from build123d import *

# Parameters (mm, degrees)
SKETCH1_R           = 28
SKETCH1_R_2         = 15
BOSS_EXTRUDE1_DEPTH = 106
SKETCH4_R           = 28
SKETCH4_R_2         = 15
BOSS_EXTRUDE2_DEPTH = 53
CUT_EXTRUDE2_START  = -106
SKETCH5_R           = 15
CUT_EXTRUDE2_DEPTH  = 106
SCALE1_SCALE        = 0.33


with BuildPart() as part:
    # Sketch1 → Boss-Extrude1 (new body)
    with BuildSketch(Plane(origin=(0, 0, 0), x_dir=(1, 0, 0), z_dir=(0, 1, 0))):
        with Locations(Location((0, 0, 0), (0, 0, 270))):
            Circle(SKETCH1_R)
        with Locations(Location((0, 0, 0), (0, 0, 270))):
            Circle(SKETCH1_R_2, mode=Mode.SUBTRACT)
    extrude(amount=BOSS_EXTRUDE1_DEPTH)

    # Sketch4 → Boss-Extrude2 (add, symmetric)
    with BuildSketch(Plane(origin=(0, 0, 0), x_dir=(0, 0, -1), z_dir=(1, 0, 0))):
        with Locations((38, 53)):
            Circle(SKETCH4_R)
        with Locations((38, 53)):
            Circle(SKETCH4_R_2, mode=Mode.SUBTRACT)
    extrude(amount=BOSS_EXTRUDE2_DEPTH, both=True)

    # Sketch5 → Cut-Extrude2 (cut)
    with BuildSketch(Plane(origin=(53, 0, 0), x_dir=(0, 0, -1), z_dir=(1, 0, 0)).offset(CUT_EXTRUDE2_START)):
        with Locations((38, 53)):
            Circle(SKETCH5_R)
    extrude(amount=CUT_EXTRUDE2_DEPTH, mode=Mode.SUBTRACT)


with BuildPart() as part_1:
    # Scale1: scaled about (-6.4e-07, 52.999995481, -18.972102588)
    add(part.part.scale(SCALE1_SCALE).moved(Location((-4.29e-07, 35.509996972, -12.711308734))))


solid = part_1.part
Build history of the part. All positions in model axes, mm. A direction names the side the tool comes from. Coordinates: 2 decimals unless noted, no trailing zeros. Write each loop counter-clockwise with the first axis right and the second up, starting at its lowest first coordinate (ties: lowest second). Pieces come first, ordered by that corner, then holes.
(1) Cut at C-C on y = 60. List the corners of the cut face in (x, z), and give its area (3 significant figures).
(2) 3-axis set-ups, long thin cutter, end or side, ignore diameter. For faces 4 (the cylindrical face through (0.05, 53.08, -16.01)), 5 (the flat face through (17.49, 49, -29)): which of +Z, -Z, +X, -X, +Y, -Y reach the whole face in a straight line?
(3) Cut at B-B on z = -15. List the corners of the cut face in (x, y).
(4) Cut at A-A on x = 2. List the corners of the cut face in (y, z), and give its area (3 significant figures).
(5) Cut at D-D on x = -7. List the corners of the cut face in (y, z).
(6) Drill centre lines: line 1 (Z direction, x = 0, y = 53); line 2 (Z direction, x = 0, y = 51.5); line 3 (Z direction, x = 5, y = 55.5). Where is each one in solid material? Low to high.
(7) Mould opens along X. For faces 1 (the cylindrical face through (2.78, 52.76, -3.9)), 2 (the cylindrical face through (1.49, 52.76, -7.99)), 3 (the flat face through (-4, 70.49, -9)) say: pulls with the +X half, pulls with the -X half, needs draft (parallel to the pull), parting line crosses it, or undercut.
(8) Pin check, flat tips, straight feed: pin 1 Ø9 at (y, z) = (53, -25.25) entering from +X; pin 2 Ø1.5 at (x, y) = (7, 51.5) entering from -Z; pin 3 Ø11.5 at (x, z) = (0, -12.71) entering from +Y; pin 4 Ø6 at (y, z) = (61, -11.5) entering from -X. Stop position of each tip, or through.
Working result:
1. outline: (-17.49, -31.28) - (17.49, -31.28) - (17.49, -19.22) - (6.56, -19.22) arc R9.24 ccw (long way) to (-6.56, -19.22) - (-17.49, -19.22) - close; hole circle Ø9.9 at (0, -12.71)
1. area: 589 mm2
2. face 4: none
2. face 5: +Z, -Z, +X, +Y, -Y
3. outline: (-8.95, 35.51) - (-4.39, 35.51) - (-4.39, 70.49) - (-8.95, 70.49) - close; (4.39, 35.51) - (8.95, 35.51) - (8.95, 70.49) - (4.39, 70.49) - close
4. outline: (35.51, -21.73) - (44.46, -21.73) arc R9.24 ccw (long way) to (61.54, -21.73) - (70.49, -21.73) - (70.49, -17.24) - (57.6, -17.24) arc R9.24 ccw to (48.4, -17.24) - (35.51, -17.24) - close; (35.51, -8.18) - (70.49, -8.18) - (70.49, -3.69) - (35.51, -3.69) - close; hole circle Ø9.9 at (53, -25.25)
4. area: 443 mm2
5. outline: (35.51, -18.74) - (46.44, -18.74) arc R9.24 ccw (long way) to (59.56, -18.74) - (70.49, -18.74) - (70.49, -6.68) - (35.51, -6.68) - close; hole circle Ø9.9 at (53, -25.25)
6. line 1: z = -34.49 to -30.2, -20.3 to -16.01, -7.76 to -3.47
6. line 2: z = -34.37 to -29.97, -20.53 to -16.13, -7.76 to -3.47
6. line 3: z = -34.15 to -29.52, -20.98 to -4.94
7. face 1: parting line crosses it
7. face 2: undercut
7. face 3: needs draft
8. pin 1: passes through
8. pin 2: stops at z = -34.46
8. pin 3: stops at y = 70.49
8. pin 4: stops at x = -9.24
